from build123d import *

# Parameters (mm, degrees)
BOSS_EXTRUDE1_DEPTH  = 25.4
BOSS_EXTRUDE7_DEPTH  = 25.4
SKETCH5_W            = 22.225
SKETCH5_H            = 22.225
BOSS_EXTRUDE10_DEPTH = 19.05
SKETCH6_W            = 22.225
SKETCH6_H            = 22.225
BOSS_EXTRUDE11_DEPTH = 19.05
SKETCH7_W            = 22.225
SKETCH7_H            = 22.225
BOSS_EXTRUDE13_DEPTH = 19.05


with BuildPart() as part:
    # Sketch1 → Boss-Extrude1 (new body)
    with BuildSketch(Plane(origin=(0, 0, 0), x_dir=(1, 0, 0), z_dir=(0, 1, 0))):
        with BuildLine():
            Line((-50.8, 0), (-27.030115421, 0))
            Line((-27.030115421, 0), (-37.735458494, -29.41268836))
            Line((-37.735458494, -29.41268836), (-13.867265926, -38.1))
            Line((-13.867265926, -38.1), (9.925939517, 27.27129469))
            Line((9.925939517, 27.27129469), (9.925939517, 38.1))
            Line((9.925939517, 38.1), (-15.474060483, 38.1))
            ThreePointArc((-15.474060483, 38.1), (-19.193804362, 29.119743879), (-28.174060483, 25.4))
            Line((-28.174060483, 25.4), (-50.8, 25.4))
            Line((-50.8, 25.4), (-50.8, 0))
        make_face()
    extrude(amount=BOSS_EXTRUDE1_DEPTH)

    # Sketch4 → Boss-Extrude7 (add)
    with BuildSketch(Plane(origin=(0, 0, -38.1), x_dir=(-1, 0, 0), z_dir=(0, 0, -1))):
        with BuildLine():
            Line((-9.925939517, 25.4), (-9.925939517, 0))
            Line((-9.925939517, 0), (-9.471788073, 0))
            ThreePointArc((-9.471788073, 0), (6.144801457, -61.168036219), (42.150474788, -113.023585695))
            Line((42.150474788, -113.023585695), (60.11098703, -95.063073453))
            ThreePointArc((60.11098703, -95.063073453), (15.474060483, 12.7), (60.11098703, 120.463073453))
            Line((60.11098703, 120.463073453), (42.150474788, 138.423585695))
            ThreePointArc((42.150474788, 138.423585695), (6.144801457, 86.568036219), (-9.471788073, 25.4))
            Line((-9.471788073, 25.4), (-9.925939517, 25.4))
        make_face()
    extrude(amount=BOSS_EXTRUDE7_DEPTH)

    # Sketch5 → Boss-Extrude10 (add)
    with BuildSketch(Plane(origin=(-90.287030241, 90.287030241, 0), x_dir=(0, 0, 1), z_dir=(-0.7071067811865479, 0.7071067811865472, 0))):
        with Locations((-50.8, 55.375369568)):
            Rectangle(SKETCH5_W, SKETCH5_H)
    extrude(amount=BOSS_EXTRUDE10_DEPTH)

    # Sketch6 → Boss-Extrude11 (add)
    with BuildSketch(Plane(origin=(-77.587030241, -77.587030241, 0), x_dir=(0, 0, 1), z_dir=(-0.7071067811865478, -0.7071067811865472, 0))):
        with Locations((-50.8, -37.414857326)):
            Rectangle(SKETCH6_W, SKETCH6_H)
    extrude(amount=BOSS_EXTRUDE11_DEPTH)

    # Sketch7 → Boss-Extrude13 (add)
    with BuildSketch(Plane.ZY.offset(50.8)):
        with Locations((-12.7, 12.7)):
            Rectangle(SKETCH7_W, SKETCH7_H)
    extrude(amount=BOSS_EXTRUDE13_DEPTH)


solid = part.part
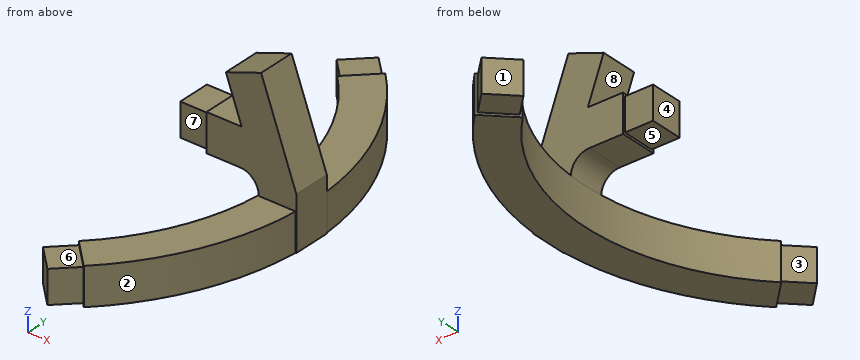
Input: part model. Units: mm. Frame: model coordinates. Face numbers are marked on the shaded views. A direction names the side the tool comes from. Give positions to 0.01 mm unless a question says otherwise; leave off trailing zeros. Write each loop counter-clockwise with the first axis right and the second up, starting at its lowest first coordinate (ties: lowest second). Pieces come first, ordered by that corner, then holes. Notation, with made-up numbers: M 73.25,-6 L 93.25,-6 A14 ccw 93.25,8 Z; hole C 4,17 d5. An arc over 180 degrees is marked long. Write item = value, one per line. Start each with the question number.
1) Draft query along Y for the marked faces 1, 2, 3 and 4. Return one class per face: +Y half, -Y half, draft (parallel to the pull), parting line (faces both ways), or undercut.
2) Cut plane A-A on x = -21. Return the cut outline in (y, z).
3) Material intervals for line 1 along Y through (x, z) = (-60, -49); line 2 along Y through (x, z) = (-64, -16); line 3 along Z through (x, y) = (-13, -44.5), sorted ascending. Write a range as [from, to].
4) Cut plane D-D on x = -2.5. Return the cut outline in (y, z), then the cut area to 3 significant figures.
5) Cut plane B-B on z = -54. Return the cut outline in (x, y).
6) Reachability of the marked faces 5, 6, 7 and 8 from +Z, -Z, +X, -X, +Y, -Y: full face, straight path, thin tool, end or side. Return the list, or none.
7) First-contact query: pin 1 Ø3 at (y, z) = (-10.5, -38) entering from -X; pin 2 Ø18 at (y, z) = (14, -8) entering from -X; pin 3 Ø12 at (y, z) = (44.5, -46.5) entering from -X. Flat tips, straight axial feed; report the tip coordinate or a pass-through.
8) Cut plane C-C on y = 56.5. Return the cut outline in (x, z).
Solved:
q1.face_1 = +Y half
q1.face_2 = -Y half
q1.face_3 = undercut
q1.face_4 = draft
q2.outline = M -87.5,-63.5 L -27.97,-63.5 L -27.97,-38.1 L -87.5,-38.1 Z; M 0,-27.62 L 25.4,-27.62 L 25.4,35.5 L 0,35.5 Z; M 53.37,-63.5 L 112.9,-63.5 L 112.9,-38.1 L 53.37,-38.1 Z
q3.line_1 = [-122.11, -97.2], [-95.17, -94.95], [120.35, 120.57], [122.6, 147.51]
q3.line_2 = [1.59, 23.81]
q3.line_3 = [-63.5, -38.1]
q4.outline = M -52.6,-63.5 L 78,-63.5 L 78,-38.1 L 25.4,-38.1 L 25.4,6.87 L 0,6.87 L 0,-38.1 L -52.6,-38.1 Z
q4.area = 4,460 mm2
q5.outline = M -72.46,-109.66 L -56.74,-125.37 L -43.27,-111.9 L -42.15,-113.02 A177.8 ccw 9.47,0 L 9.93,0 L 9.93,25.4 L 9.47,25.4 A177.8 ccw -42.15,138.42 L -43.27,137.3 L -56.74,150.77 L -72.46,135.06 L -58.99,121.59 L -60.11,120.46 A152.4 cw -60.11,-95.06 L -58.99,-96.19 Z
q6.face_5 = -Z, -X, +Y, -Y
q6.face_6 = +Z, -X, -Y
q6.face_7 = +Z, -Z, -X, -Y
q6.face_8 = -X, +Y, -Y
q7.pin_1 = -17.49
q7.pin_2 = -69.85
q7.pin_3 = -20.24
q8.outline = M -21.9,-63.5 L 4.45,-63.5 L 4.45,-38.1 L -21.9,-38.1 Z
